Job drawing, mm, ordinate dimensions from the low corner. One solid piece. Coordinates: 2 decimals unless noted, no trailing zeros. Order: outer loops, then holes, each group sorted by start corner. A loop starts at its lowest first (then second) coordinate and runs counter-clockwise, first axis right, second up. Notation, with made-up numbers: (-28.75, 64) - (2.25, 64) arc R15 cw to (2.25, 77) - close; hole circle Ø7 at (48, 74). An arc over 180 degrees is marked (long way). Write each question's results on one line, items separated by ' | '. Start each with the question number.
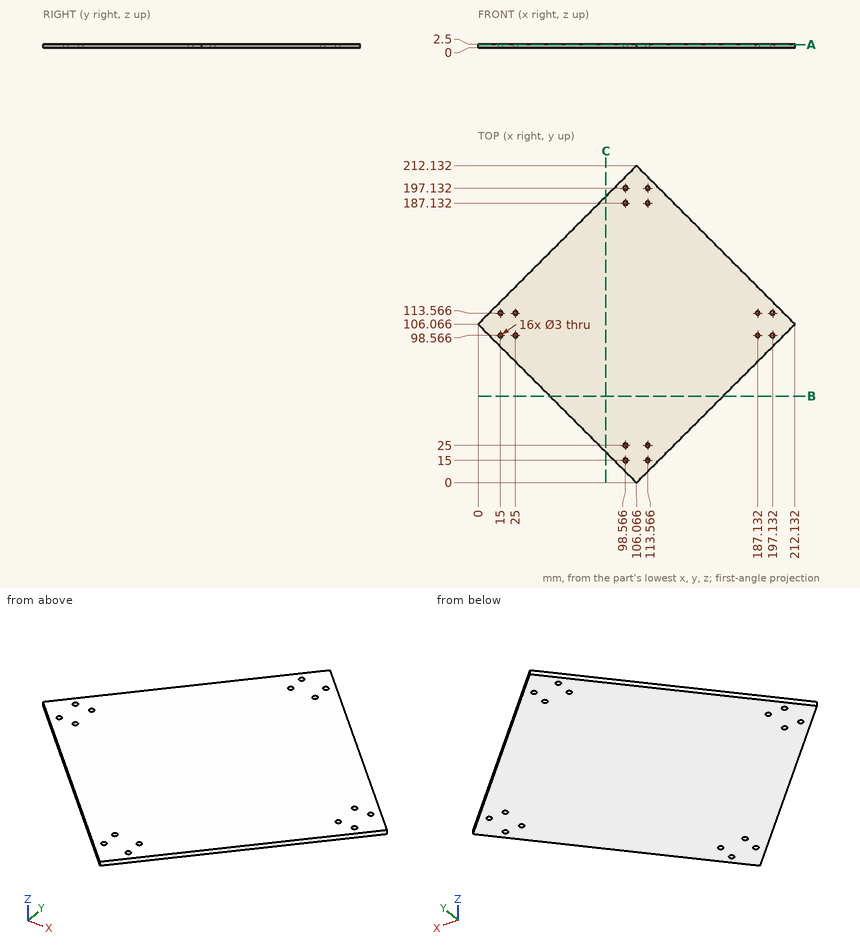
Item 1: Slice it at A-A (z = 2). Count the separate pieces of the cut face and the enclosed holes in it, then the cut area to 3 significant figures.
Item 2: Slice it at B-B (y = 58). Write the cut outline in (x, z).
Item 3: Probe probe 1 along X at (y, z) = (196, 1); probe 2 along Y at (x, z) = (26, 1.25); probe 3 along Y at (x, z) = (198, 1.8). List the from-to ranges inside material, lowest first.
Item 4: Flat gauge pins, fed straight in: P1, Ø1.5, axis at x = 184, z = 1.5, coming from the +Y side; P2, Ø1, axis at y = 89, z = 1.5, coming from the +X side. Where does each tip first touch, or does it go through?
Item 5: Slice it at C-C (x = 85.5). Write the cut outline in (y, z), then the cut area to 4 significant figures.
Resolved:
1) separate pieces: 1 | enclosed holes: 16 | area: 22,400 mm^2
2) outline: (48.07, 0) - (164.07, 0) - (164.07, 2.5) - (48.07, 2.5) - close
3) probe 1: 89.93 to 97.58, 99.55 to 112.58, 114.55 to 122.2 | probe 2: 80.07 to 97.45, 99.68 to 112.45, 114.68 to 132.07 | probe 3: 91.93 to 97.34, 99.79 to 112.34, 114.79 to 120.2
4) P1: y = 134.95 | P2: x = 195.57
5) outline: (20.57, 0) - (191.57, 0) - (191.57, 2.5) - (20.57, 2.5) - close | area: 427.5 mm^2
